Source: CAD feature listing. Evaluate the final solid. Frame: model axes, mm. A direction names the side the tool comes from. Coordinates: 2 decimals unless noted, no trailing zeros. Write each loop counter-clockwise with the first axis right and the second up, starting at its lowest first coordinate (ties: lowest second). Pieces come first, ordered by that corner, then holes. Notation, with made-up numbers: (32, 81.25) - (50, 81.25) arc R22 cw to (50, 90.25) - close; hole circle Ø9 at (70.25, 62.25). An arc over 180 degrees is marked (long way). One line per question, with ' | ' between items.
from build123d import *

# Parameters (mm, degrees)
F0_W      = 95
F0_H      = 78
F1_DEPTH  = 4
F2_W      = 70
F2_H      = 51
F3_DEPTH  = 1
F4_W      = 93
F4_H      = 76
F4_W_2    = 70
F4_H_2    = 51
F5_DEPTH  = 2
F6_W      = 70
F6_H      = 51
F7_DEPTH  = 1
F8_R      = 13
F9_DEPTH  = 1
F10_W     = 3
F10_H     = 3
F11_DEPTH = 10


with BuildPart() as f1:
    # F0 (on Front) → F1 (new body)
    with BuildSketch(Plane.XZ):
        Rectangle(F0_W, F0_H)
    extrude(amount=F1_DEPTH)

    # F2 (on face) → F3 (cut)
    with BuildSketch(Plane(origin=(0, 0, 0), x_dir=(-1, 0, 0), z_dir=(0, 1, 0))):
        Rectangle(F2_W, F2_H)
    extrude(amount=-F3_DEPTH, mode=Mode.SUBTRACT)

    # F4 (on face) → F5 (cut)
    with BuildSketch(Plane(origin=(0, 0, 0), x_dir=(-1, 0, 0), z_dir=(0, 1, 0))):
        Rectangle(F4_W, F4_H)
        Rectangle(F4_W_2, F4_H_2, mode=Mode.SUBTRACT)
    extrude(amount=-F5_DEPTH, mode=Mode.SUBTRACT)

    # F6 (on face) → F7 (cut)
    with BuildSketch(Plane.XZ.offset(4)):
        Rectangle(F6_W, F6_H)
    extrude(amount=-F7_DEPTH, mode=Mode.SUBTRACT)

    # F8 (on face) → F9 (join)
    with BuildSketch(Plane(origin=(0, -1, 0), x_dir=(-1, 0, 0), z_dir=(0, 1, 0))):
        Circle(F8_R)
    extrude(amount=F9_DEPTH)

    # F10 (on face) → F11 (join)
    with BuildSketch(Plane(origin=(0, 0, 0), x_dir=(-1, 0, 0), z_dir=(0, 1, 0))):
        Rectangle(F10_W, F10_H)
    extrude(amount=F11_DEPTH)


solid = f1.part
Item 1: Ray query, line 1 along Z through (x, y) = (16.5, -1.75); line 2 along X through (y, z) = (-0.25, -6); line 3 along Z through (x, y) = (2, -0.5). Return the intervals inside material, ascending. Write a range as [from, to].
Check sheet entries:
line 1: [-39, -38], [-25.5, 25.5], [38, 39] | line 2: [-47.5, -46.5], [-11.53, 11.53], [46.5, 47.5] | line 3: [-39, -38], [-12.85, 12.85], [38, 39]
Item 2: Pin query (flat end, axial travel): pin 1 Ø0.9 at (x, y) = (-0.5, 6) entering from +Z; pin 2 Ø3.5 at (y, z) = (5.5, -0.5) entering from -X; pin 3 Ø3.5 at (y, z) = (3, 0.5) entering from +X; pin 4 Ø8 at (y, z) = (1.5, -27.5) entering from -X. Return the tip coordinate at first contact, or that it passes through.
Check sheet entries:
pin 1: z = 1.5 | pin 2: x = -1.5 | pin 3: x = 1.5 | pin 4: x = -47.5
Item 3: Mould query, pull axis Z, two halves, no side actions, for faces 1 (the face through (1, -1, -38)), 2 (the face through (-1, -4, 27)), 3 (the face through (0, 5, -1.5)), 4 (the face through (1, -2, 26)). Classes: pulls with the +Z half, pulls with the -Z half, needs draft (parallel to the pull), parting line crosses it, or undercut.
Check sheet entries:
face 1: undercut | face 2: needs draft | face 3: pulls with the -Z half | face 4: undercut
Item 4: Cut plane A-A on z = 0. Return loops of the section in (x, y).
Check sheet entries:
outline: (-47.5, -4) - (-35, -4) - (-35, -3) - (35, -3) - (35, -4) - (47.5, -4) - (47.5, 0) - (46.5, 0) - (46.5, -2) - (35, -2) - (35, -1) - (13, -1) - (13, 0) - (1.5, 0) - (1.5, 10) - (-1.5, 10) - (-1.5, 0) - (-13, 0) - (-13, -1) - (-35, -1) - (-35, -2) - (-46.5, -2) - (-46.5, 0) - (-47.5, 0) - close
Item 5: Cut plane D-D on z = -31. Return loops of the section in (x, y).
Check sheet entries:
outline: (-47.5, -4) - (47.5, -4) - (47.5, 0) - (46.5, 0) - (46.5, -2) - (-46.5, -2) - (-46.5, 0) - (-47.5, 0) - close
Item 6: Access query for faces 5 (the face through (0, -3, 0)), 6 (the face through (1, -1, 38)), 7 (the face through (-1.5, 5, 0)). Directions: +Z, -Z, +X, -X, +Y, -Y. A direction counts if a zero-diameter tool reaches every point of the face in a straight line with its end or side. Return the directions, or none.
Check sheet entries:
face 5: -Y | face 6: +Y | face 7: +Z, -Z, -X, +Y
Item 7: Cut plane B-B on x = 31.5. Return loops of the section in (y, z), and give its area (3 significant figures).
Check sheet entries:
outline: (-4, -39) - (0, -39) - (0, -38) - (-2, -38) - (-2, -25.5) - (-1, -25.5) - (-1, 25.5) - (-2, 25.5) - (-2, 38) - (0, 38) - (0, 39) - (-4, 39) - (-4, 25.5) - (-3, 25.5) - (-3, -25.5) - (-4, -25.5) - close | area: 160 mm²
Item 8: Cut plane C-C on y = 4.25. Return loops of the section in (x, z), and give its area (3 significant figures).
Check sheet entries:
outline: (-1.5, -1.5) - (1.5, -1.5) - (1.5, 1.5) - (-1.5, 1.5) - close | area: 9.00 mm²
